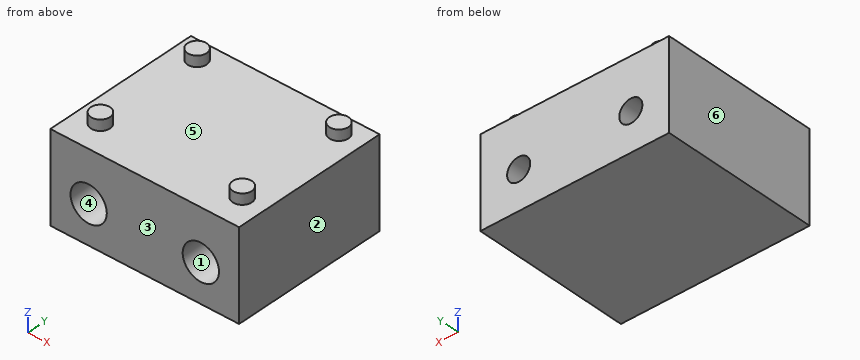
```python
from build123d import *

# Parameters (mm, degrees)
SKETCH015_W     = 28.6
SKETCH015_H     = 13.55
SKETCH015_R     = 1.75
PAD007_DEPTH    = 24
SKETCH016_R     = 2.75
POCKET008_DEPTH = 8
SKETCH017_R     = 1.45
PAD008_DEPTH    = 1.6


with BuildPart() as part:
    # Sketch015 (on Face21 of Binder004) → Pad007 (new body)
    with BuildSketch(Plane.XZ.offset(-32.95)):
        with Locations((13.74978, -6.775)):
            Rectangle(SKETCH015_W, SKETCH015_H)
        with Locations((5.24978, -7.7)):
            Circle(SKETCH015_R, mode=Mode.SUBTRACT)
        with Locations((22.24978, -7.7)):
            Circle(SKETCH015_R, mode=Mode.SUBTRACT)
    extrude(amount=PAD007_DEPTH)

    # Sketch016 (on Face8 of Pad007) → Pocket008 (cut)
    with BuildSketch(Plane.XZ.offset(-8.95)):
        with Locations((5.24978, -7.7)):
            Circle(SKETCH016_R)
        with Locations((22.24978, -7.7)):
            Circle(SKETCH016_R)
    extrude(amount=-POCKET008_DEPTH, mode=Mode.SUBTRACT)

    # Sketch017 (on Face6 of Pocket008) → Pad008 (join)
    with BuildSketch(Plane.XY):
        with Locations((3, 13.5)):
            Circle(SKETCH017_R)
        with Locations((24.5, 13.5)):
            Circle(SKETCH017_R)
        with Locations((24.5, 30)):
            Circle(SKETCH017_R)
        with Locations((3, 30)):
            Circle(SKETCH017_R)
    extrude(amount=PAD008_DEPTH)


solid = part.part
```
Verification items for the finished model (mm, model axes). Face numbers are marked on the shaded views. A direction names the side the tool comes from. Coordinates: 2 decimals unless noted, no trailing zeros. Write each loop counter-clockwise with the first axis right and the second up, starting at its lowest first coordinate (ties: lowest second). Pieces come first, ordered by that corner, then holes. Notation, with made-up numbers: (17.25, -13.75) - (68.25, -13.75) arc R19 ccw to (68.25, 4.25) - close; hole circle Ø9 at (-22, 0.25). An arc over 180 degrees is marked (long way). One line per question, with ' | ' between items. Start each with the question number.
1. Section check D-D (x = 3). Enter the section's corners in (y, z), plus the area to 3 significant figures.
2. Material ranges on line 1 along X through (y, z) = (29, -7.7); line 2 along X through (y, z) = (31, -8.75); line 3 along Z through (x, y) = (22.25, 25), recorded low to high.
3. Gauge pin test, flat ends, axial feed: P1, Ø2.5, axis at x = 5.5, z = -8, coming from the -Y side; P2, Ø4, axis at x = 8.5, y = 24, coming from the +Z side. Record the tip position at first contact, or that the pin passes through.
4. Section check A-A (z = -7.7). Enter the section's corners in (x, y).
5. Section check C-C (x = 6.25). Enter the section's corners in (y, z), plus the area to 3 significant figures.
6. Section check B-B (y = 24.25). Enter the section's corners in (x, z), plus the area to 3 significant figures.
7. Access from +Z, -Z, +X, -X, +Y, -Y to the whole of each face (thin tool, end or side, straight path). Record for the marked faces 4, 5 and 6.
8. Draft check along X on the marked faces 1, 2 and 3. Enter one of: released by +X, released by -X, zero draft, split by the parting line, or undercut.
Computed values:
1) outline: (8.95, -13.55) - (32.95, -13.55) - (32.95, 0) - (31.45, 0) - (31.45, 1.6) - (28.55, 1.6) - (28.55, 0) - (14.95, 0) - (14.95, 1.6) - (12.05, 1.6) - (12.05, 0) - (8.95, 0) - (8.95, -6.12) - (16.95, -6.12) - (16.95, -9.28) - (8.95, -9.28) - close | area: 309 mm²
2) line 1: -0.55 to 3.5, 7 to 20.5, 24 to 28.05 | line 2: -0.55 to 3.85, 6.65 to 20.85, 23.65 to 28.05 | line 3: -13.55 to -9.45, -5.95 to 0
3) P1: through | P2: z = 0
4) outline: (-0.55, 8.95) - (2.5, 8.95) - (2.5, 16.95) - (3.5, 16.95) - (3.5, 32.95) - (-0.55, 32.95) - close; (7, 16.95) - (8, 16.95) - (8, 8.95) - (19.5, 8.95) - (19.5, 16.95) - (20.5, 16.95) - (20.5, 32.95) - (7, 32.95) - close; (24, 16.95) - (25, 16.95) - (25, 8.95) - (28.05, 8.95) - (28.05, 32.95) - (24, 32.95) - close
5) outline: (8.95, -13.55) - (32.95, -13.55) - (32.95, -9.14) - (16.95, -9.14) - (16.95, -10.26) - (8.95, -10.26) - close; (8.95, -5.14) - (16.95, -5.14) - (16.95, -6.26) - (32.95, -6.26) - (32.95, 0) - (8.95, 0) - close | area: 238 mm²
6) outline: (-0.55, -13.55) - (28.05, -13.55) - (28.05, 0) - (-0.55, 0) - close; hole circle Ø3.5 at (5.25, -7.7); hole circle Ø3.5 at (22.25, -7.7) | area: 368 mm²
7) face 4: -Y | face 5: +Z | face 6: +Z, -Z, -X, +Y, -Y
8) face 1: undercut | face 2: released by +X | face 3: zero draft
